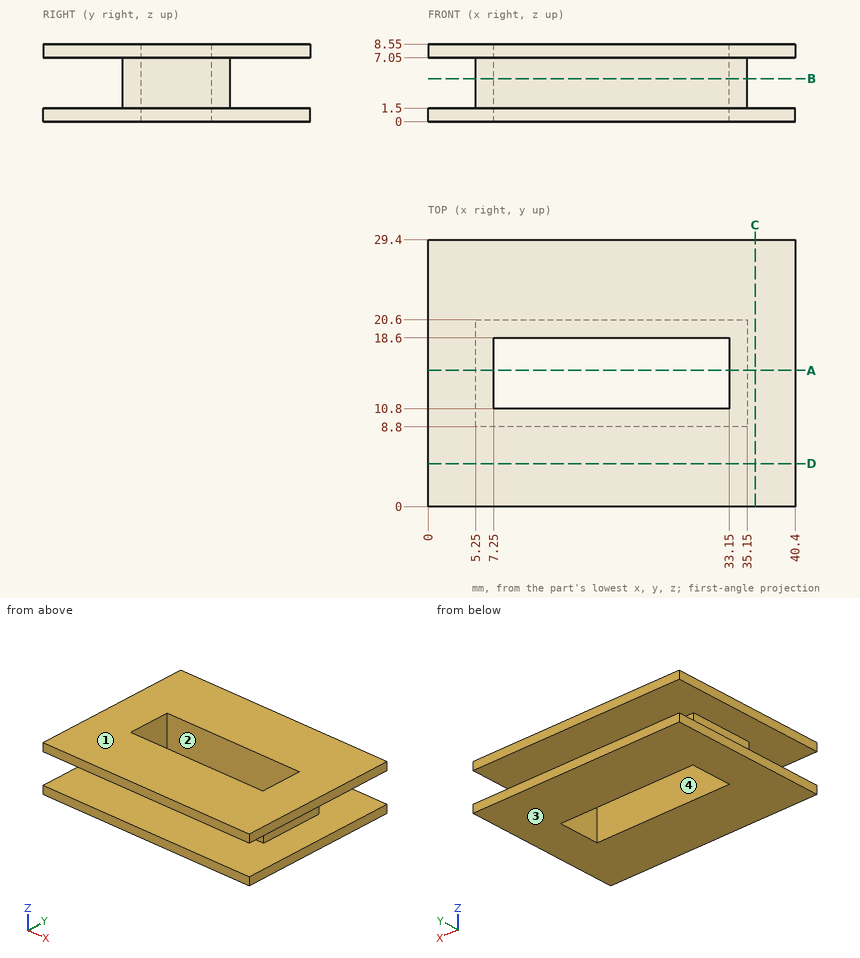
Design review of the part shown in the three views and the two pictorial views. Dimensions are in mm from the part's minimum x, y and z. A direction names the side the tool comes from. Round coordinates to 2 decimals unless told otherwise and drop trailing zeros. Loops run counter-clockwise (first coordinate to the right, second up) from the corner with the lowest first, then second, coordinate; pieces in that order, holes last.
Q1. Insertion check: pin 1 Ø1.7 at (y, z) = (16.5, 4.5) entering from -X; pin 2 Ø1.7 at (x, z) = (25.5, 4.5) entering from -Y; pin 3 Ø3 at (x, z) = (14.5, 4) entering from +Y; pin 4 Ø3 at (y, z) = (23, 3.5) entering from -X. Each pin has a flat end and moves straight along its axis. Give the tip position at first contact, or say it passes through.
Result sheet:
pin 1: stops at x = 5.25
pin 2: stops at y = 8.8
pin 3: stops at y = 20.6
pin 4: passes through
Q2. Machinability: for the marked faces 1 and 2, which of the approach directions +Z, -Z, +X, -X, +Y, -Y give a long, thin tool a straight path to every point of the face, cutting with its end or side? Answer none if there is none.
Result sheet:
face 1: +Z, +X, -X, +Y, -Y
face 2: +Z, -Z
Q3. Mouldability with a two-part tool opening along Y and no side actions: class the marked faces 3 and 4 as +Y half, -Y half, draft (parallel to the pull), parting line (faces both ways), or undercut.
Result sheet:
face 3: draft
face 4: undercut
Q4. Add section A-A on y = 15. Write out the cut boundary in (x, z).
Result sheet:
outline: (0, 0) - (7.25, 0) - (7.25, 8.55) - (0, 8.55) - (0, 7.05) - (5.25, 7.05) - (5.25, 1.5) - (0, 1.5) - close; (33.15, 0) - (40.4, 0) - (40.4, 1.5) - (35.15, 1.5) - (35.15, 7.05) - (40.4, 7.05) - (40.4, 8.55) - (33.15, 8.55) - close
Q5. Add section B-B on z = 4.75. Write out the cut boundary in (x, y), plus the area to 3 significant figures.
Result sheet:
outline: (5.25, 8.8) - (35.15, 8.8) - (35.15, 20.6) - (5.25, 20.6) - close; hole (7.25, 10.8) - (33.15, 10.8) - (33.15, 18.6) - (7.25, 18.6) - close
area: 151 mm2
Q6. To check wall thickness, follow line 1 along Z through (x, y) = (3.5, 19.25); line 2 along Y through (x, z) = (25, 2.5); line 3 along Y through (x, z) = (32, 0.75). State the ranges of each line that lie inside material, in increasing order.
Result sheet:
line 1: z = 0 to 1.5, 7.05 to 8.55
line 2: y = 8.8 to 10.8, 18.6 to 20.6
line 3: y = 0 to 10.8, 18.6 to 29.4
Q7. Add section C-C on x = 36. Write out the cut boundary in (y, z).
Result sheet:
outline: (0, 0) - (29.4, 0) - (29.4, 1.5) - (0, 1.5) - close; (0, 7.05) - (29.4, 7.05) - (29.4, 8.55) - (0, 8.55) - close
Q8. Add section D-D on y = 4.75. Write out the cut boundary in (x, z), plus the area to 3 significant figures.
Result sheet:
outline: (0, 0) - (40.4, 0) - (40.4, 1.5) - (0, 1.5) - close; (0, 7.05) - (40.4, 7.05) - (40.4, 8.55) - (0, 8.55) - close
area: 121 mm2
